Answer from the drawing. Dimensions are ordinates in mm from the lowest x, y and z of the part. A direction names the side the tool comes from. Coordinates: 2 decimals unless noted, no trailing zeros. Write each loop counter-clockwise with the first axis right and the second up, starting at its lowest first coordinate (ties: lowest second). Pieces come first, ordered by that corner, then holes. Notation, with made-up numbers: (6.5, 51.5) -> (56.5, 51.5) arc R26 cw to (56.5, 85.5) -> close; hole circle Ø11 at (15.5, 61.5). An arc over 180 degrees is marked (long way). Return JSON: item names as keys, results as strings.
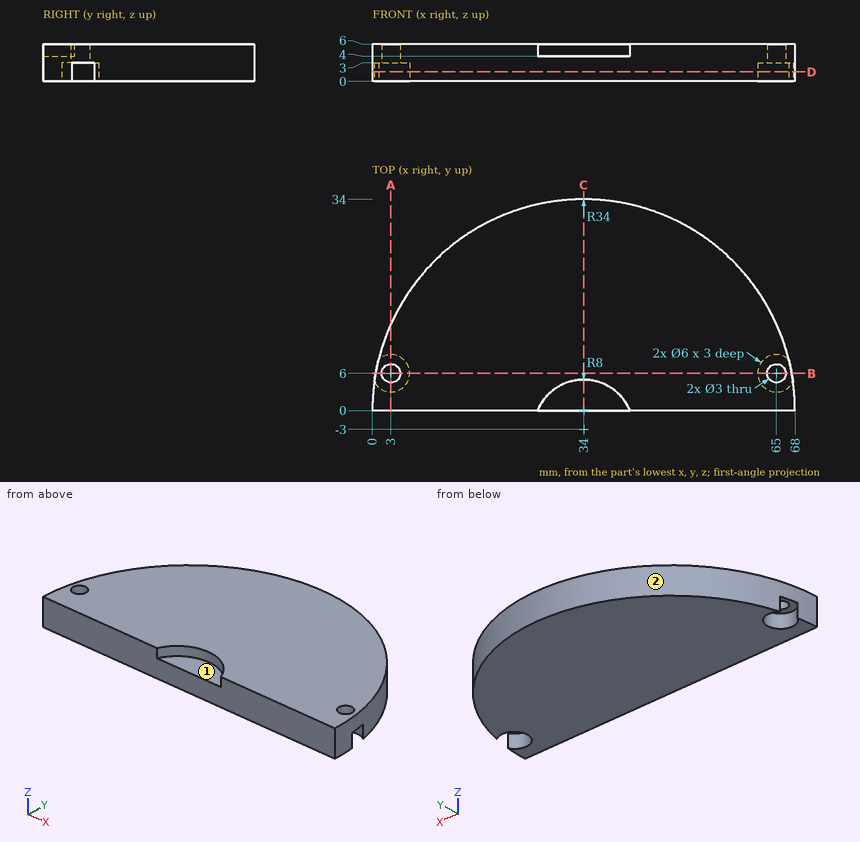
1. The part is cut by section B-B (y = 6). Determine the outline of the cut face in (x, z), then the cut area to 3 significant figures.
Taken from the geometry:
{"outline": "(0.53, 3) -> (1.5, 3) -> (1.5, 6) -> (0.53, 6) -> close; (4.5, 3) -> (6, 3) -> (6, 0) -> (62, 0) -> (62, 3) -> (63.5, 3) -> (63.5, 6) -> (4.5, 6) -> close; (66.5, 3) -> (67.47, 3) -> (67.47, 6) -> (66.5, 6) -> close", "area": "351 mm2"}
2. The part is cut by section C-C (x = 34). Determine the outline of the cut face in (y, z), then the cut area to 3 significant figures.
Taken from the geometry:
{"outline": "(0, 0) -> (34, 0) -> (34, 6) -> (5, 6) -> (5, 4) -> (0, 4) -> close", "area": "194 mm2"}
3. Consider L1, parallel to X at y = 6, z = 5.1; L2, parallel to Y at x = 3, z = 1.55; L3, parallel to X at y = 6, z = 2.1. Determine where each line is inside the solid, lowest interval first.
Taken from the geometry:
{"L1": "x = 0.53 to 1.5, 4.5 to 63.5, 66.5 to 67.47", "L2": "y = 0 to 3, 9 to 13.96", "L3": "x = 6 to 62"}
4. Flat-ended cylindrical pins translate along their axes: pin 1 Ø3 at (x, z) = (49.5, 0.5) entering from +Y; pin 2 Ø1.5 at (x, z) = (19.5, 1) entering from +Y; pin 3 Ø3 at (y, z) = (6, 3.5) entering from -X. Find the tip coordinate at first contact, or state that the pin passes through.
Taken from the geometry:
{"pin 1": "stops at y = 30.98", "pin 2": "stops at y = 31.1", "pin 3": "stops at x = 0.3"}
5. The part is cut by section D-D (z = 1.5). Determine the outline of the cut face in (x, y).
Taken from the geometry:
{"outline": "(0, 0) -> (68, 0) arc R34 ccw to (67.68, 4.65) arc R3 cw (long way) to (66.98, 8.25) arc R34 ccw to (1.02, 8.25) arc R3 cw (long way) to (0.32, 4.65) arc R34 ccw to start"}
6. A tool of negligible diameter and unlimited length cuts with its end or side. For the marked faces 1 and 2, from which of +Z, -Z, +X, -X, +Y, -Y can it reach the whole face along a straight path? Write none if from no direction.
Taken from the geometry:
{"face 1": "+Z, -Y", "face 2": "+Z, -Z, +Y"}
7. The part is cut by section A-A (x = 3). Determine the outline of the cut face in (y, z), then the cut area to 3 significant figures.
Taken from the geometry:
{"outline": "(0, 0) -> (3, 0) -> (3, 3) -> (4.5, 3) -> (4.5, 6) -> (0, 6) -> close; (7.5, 3) -> (9, 3) -> (9, 0) -> (13.96, 0) -> (13.96, 6) -> (7.5, 6) -> close", "area": "56.8 mm2"}
